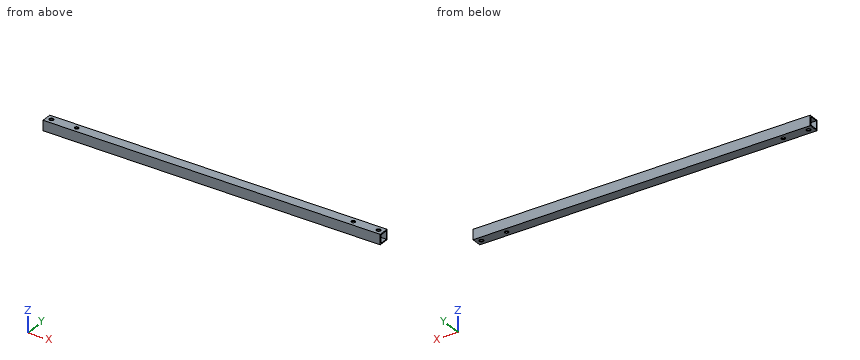
from build123d import *

# Parameters (mm, degrees)
SKETCH_1_W          = 10
SKETCH_1_H          = 10
SKETCH_1_W_2        = 8
SKETCH_1_H_2        = 8
EXTRUDE_1_DEPTH     = 333.544819152
SKETCH_2_R          = 2.1
SKETCH_2_R_2        = 2
CUT_EXTRUDE_1_DEPTH = 334.732147662


with BuildPart() as part:
    # ｽｹｯﾁ1 → 押し出し-薄板1 (new body)
    with BuildSketch(Plane(origin=(0, 0, 0), x_dir=(0, -1, 0), z_dir=(1, 0, 0))):
        Rectangle(SKETCH_1_W, SKETCH_1_H)
        Rectangle(SKETCH_1_W_2, SKETCH_1_H_2, mode=Mode.SUBTRACT)
    extrude(amount=EXTRUDE_1_DEPTH)

    # ｽｹｯﾁ2 → ｶｯﾄ - 押し出し1 (cut, through all)
    with BuildSketch(Plane.XY.offset(5)):
        with Locations((5, 0)):
            Circle(SKETCH_2_R)
        with Locations(Location((328.544819152, 0, 0), (0, 0, 180))):
            Circle(SKETCH_2_R)
        with Locations((30, 0)):
            Circle(SKETCH_2_R_2)
        with Locations(Location((303.544819152, 0, 0), (0, 0, 180))):
            Circle(SKETCH_2_R_2)
    extrude(amount=-CUT_EXTRUDE_1_DEPTH, mode=Mode.SUBTRACT)


solid = part.part
The model under review builds one solid part; all positions refer to its coordinate system, in mm. Round coordinates to 2 decimals unless told otherwise and drop trailing zeros. Loops run counter-clockwise (first coordinate to the right, second up) from the corner with the lowest first, then second, coordinate; pieces in that order, holes last. Notation, with made-up numbers: (-30, 64) -> (-1, 64) arc R23 ccw to (-1, 74) -> close; hole circle Ø5 at (24, -22). An arc over 180 degrees is marked (long way). Write item = value, one per line. Start each with the question number.
Item 1: To check wall thickness, follow L1, parallel to Z at x = 232.5, y = 2; L2, parallel to Y at x = 30, z = 4.65; L3, parallel to Y at x = 5, z = -4.7. State the ranges of each line that lie inside material, in increasing order.
Item 2: Take a section at C-C on y = 0. Count the separate pieces of the cut face and the enclosed holes in it, plus the area to 3 significant figures.
Item 3: Take a section at A-A on z = -1.75. Give the boundary of the cut face in (x, y), plus the area to 3 significant figures.
Item 4: Take a section at B-B on x = 69.5. Give the boundary of the cut face in (y, z).
Item 5: Insertion check: pin 1 (5.5 mm diameter, centred on x = 5, y = 0, fed in from +Z). The pin has a flat end and moves straight along its axis. Give the tip position at first contact, or say it passes through.
Result:
q1.L1 = -5 to -4, 4 to 5
q1.L2 = -5 to -2, 2 to 5
q1.L3 = -5 to -2.1, 2.1 to 5
q2.separate_pieces = 10
q2.enclosed_holes = 0
q2.area = 634 mm²
q3.outline = (0, -5) -> (333.54, -5) -> (333.54, -4) -> (0, -4) -> close; (0, 4) -> (333.54, 4) -> (333.54, 5) -> (0, 5) -> close
q3.area = 667 mm²
q4.outline = (-5, -5) -> (5, -5) -> (5, 5) -> (-5, 5) -> close; hole (-4, -4) -> (4, -4) -> (4, 4) -> (-4, 4) -> close
q5.pin_1 = 5
